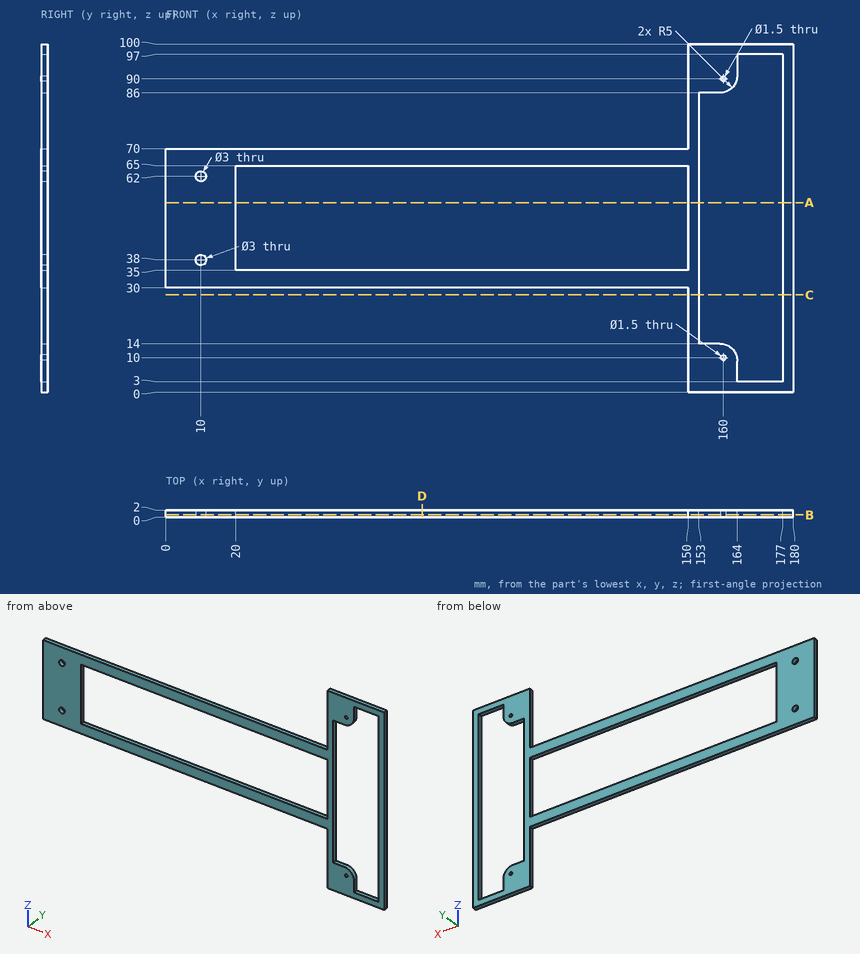
For this review, use the dimensioned drawing (mm, ordinates from the lowest corner) and the shaded views. Coordinates: 2 decimals unless noted, no trailing zeros. Write each loop counter-clockwise with the first axis right and the second up, starting at its lowest first coordinate (ties: lowest second). Pieces come first, ordered by that corner, then holes. Notation, with made-up numbers: (0.25, 56) - (14.25, 56) arc R13 ccw to (14.25, 76) - close; hole circle Ø8 at (22.25, 24.25). An arc over 180 degrees is marked (long way). Answer in a Markdown table with one row per item. Add a question column.
Q1. Clearance check with flat-ended pins moving along their axes: pin 1 (2.5 mm diameter, centred on x = 160, z = 10, fed in from +Y); pin 2 (2.5 mm diameter, centred on x = 10, z = 38, fed in from -Y); pin 3 (1 mm diameter, centred on y = 0.5, z = 83, fed in from -X). State where each tip first meets the part, or that it passes through.
Q2. To check wall thickness, follow line 1 along Z through (x, y) = (10, 1.05); line 2 along X through (y, z) = (0.7, 54.5); line 3 along Z through (x, y) = (78.5, 1). State the ranges of each line that lie inside material, in increasing order. Write a range as from..to.
Q3. Consider section B-B on y = 0.7. Give the boundary of the cut face in (x, z), then the cut area to 3 significant figures.
Q4. Consider section D-D on x = 73.5. Give the boundary of the cut face in (y, z).
Q5. Consider section A-A on z = 54.5. Give the boundary of the cut face in (x, y), then the cut area to 3 significant figures.
Q6. Consider section C-C on z = 28. Give the boundary of the cut face in (x, y), then the cut area to 3 significant figures.
Answers below:
| question | item | result |
|---|---|---|
| 1 | pin 1 | y = 2 |
| 1 | pin 2 | through |
| 1 | pin 3 | x = 150 |
| 2 | line 1 | 30..36.5, 39.5..60.5, 63.5..70 |
| 2 | line 2 | 0..20, 150..153, 177..180 |
| 2 | line 3 | 30..35, 65..70 |
| 3 | outline | (0, 30) - (150, 30) - (150, 0) - (180, 0) - (180, 100) - (150, 100) - (150, 70) - (0, 70) - close; hole circle Ø3 at (10, 38); hole circle Ø3 at (10, 62); hole (20, 35) - (150, 35) - (150, 65) - (20, 65) - close; hole (153, 14) - (159, 14) arc R5 cw to (164, 9) - (164, 3) - (177, 3) - (177, 97) - (164, 97) - (164, 91) arc R5 cw to (159, 86) - (153, 86) - close; hole circle Ø1.5 at (160, 10); hole circle Ø1.5 at (160, 90) |
| 3 | area | 3,060 mm² |
| 4 | outline | (0, 30) - (2, 30) - (2, 35) - (0, 35) - close; (0, 65) - (2, 65) - (2, 70) - (0, 70) - close |
| 5 | outline | (0, 0) - (20, 0) - (20, 2) - (0, 2) - close; (150, 0) - (153, 0) - (153, 2) - (150, 2) - close; (177, 0) - (180, 0) - (180, 2) - (177, 2) - close |
| 5 | area | 52.0 mm² |
| 6 | outline | (150, 0) - (153, 0) - (153, 2) - (150, 2) - close; (177, 0) - (180, 0) - (180, 2) - (177, 2) - close |
| 6 | area | 12.0 mm² |
